Geometry check sheet. Reference: the model listing, model coordinates, mm. A direction names the side the tool comes from. Give positions to 0.01 mm unless a question says otherwise; leave off trailing zeros. Write each loop counter-clockwise with the first axis right and the second up, starting at its lowest first coordinate (ties: lowest second). Pieces come first, ordered by that corner, then holes. Notation, with made-up numbers: M 43,16 L 69,16 A20 cw 69,42 Z; hole C -6,31.25 d4. An arc over 180 degrees is marked long. Use one line per item in the form item = value. Start each with the question number.
Autodesk Inventor part; units mm, degrees
ref_plane "YZ Plane" through (0, 0, 0) normal (1, 0, 0) x (0, 1, 0)
ref_plane "XZ Plane" through (0, 0, 0) normal (0, 1, 0) x (-1, 0, 0)
ref_plane "XY Plane" through (0, 0, 0) normal (0, 0, 1) x (1, 0, 0)
sketch "Sketch1" plane through (0, 0, 0) normal (0, 0, 1) x (1, 0, 0)
  line L0 (0, 0) -> (25.4, 0)
  line L1 (25.4, 0) -> (25.4, 25.4)
  line L2 (25.4, 25.4) -> (0, 25.4)
  line L3 (0, 25.4) -> (0, 0)
  line L4 (1.5875, 23.8125) -> (23.8125, 23.8125)
  line L5 (23.8125, 23.8125) -> (23.8125, 1.5875)
  line L6 (23.8125, 1.5875) -> (1.5875, 1.5875)
  line L7 (1.5875, 1.5875) -> (1.5875, 23.8125)
  dimension "d0" = 25.4
  dimension "d2" = 25.4
  dimension "d3" = 1.5875
extrude "Extrusion1" add sketch "Sketch1" along normal blind 596.9
sketch "Sketch3" plane through (0, 0, 0) normal (0, -1, 0) x (1, 0, 0)
  circle A0 centre (12.7, 574.675) radius 3.3782
  circle A1 centre (12.7, 542.925) radius 3.3782
extrude "Extrusion3" cut sketch "Sketch3" against normal blind 25.4
sketch "Sketch4" plane through (0, 0, 0) normal (-1, 0, 0) x (0, 0, 1)
  circle A0 centre (533.4, 12.7) radius 3.3782
  circle A1 centre (584.2, 12.7) radius 3.3782
extrude "Extrusion4" cut sketch "Sketch4" against normal blind 25.4
sketch "Sketch5" plane through (25.4, 0, 0) normal (1, 0, 0) x (0, 0, -1)
  line L0 (0, 25.4) -> (-596.9, 25.4)
  line L1 (-596.9, 0) -> (-596.9, 25.4)
  circle A0 centre (-498.475, 12.7) radius 3.3782
  circle A1 centre (-304.8, 12.7) radius 3.3782
  circle A2 centre (-114.3, 12.7) radius 3.3782
  dimension "d12" = 6.7564
  dimension "d13" = 6.7564
  dimension "d14" = 98.425
  dimension "d15" = 292.1
  dimension "d16" = 6.7564
  dimension "d17" = 482.6
  dimension "d18" = 12.7
  dimension "d19" = 12.7
  dimension "d20" = 12.7
extrude "Extrusion5" cut sketch "Sketch5" against normal blind 25.4
properties part number "Inner Mount" material "Aluminum 6061"
(1) Depth check by flat-ended pin: pin 1 (12 mm diameter, centred on y = 21.5, z = 529.5, fed in from -X). Enter the tip coordinate at first touch or a pass-through.
(2) Draft check along Y on faces 3 (the flat face through (13, 0, 294)), 4 (the flat face through (1, 13, 596.9)), 5 (the flat face through (13, 23.812, 294)). Enter one of: released by +Y, released by -Y, zero draft, split by the parting line, or undercut.
(3) Sectioned sample at A-A, the plane x = 5.5. Record the boundary of the cut face in (y, z), plus the area to 3 significant figures.
(4) Tool access check on faces 1 (the flat face through (0, 13, 294)), 2 (the flat face through (23.812, 13, 294)). Record the directions out of +Z, -Z, +X, -X, +Y, -Y that give a thin tool (end or side, any length) a straight path to the whole face; none if there is none.
(5) Sectioned sample at B-B, the plane z = 358.5. Record the boundary of the cut face in (x, y).
(6) Thickness scan on probe 1 along Y at (x, z) = (3.5, 359); probe 2 along Z at (x, y) = (12.7, 0.45). Record the ranges inside material, lowest first. Write a range as [from, to].
Numbers:
q1.pin_1 = 0
q2.face_3 = released by -Y
q2.face_4 = zero draft
q2.face_5 = undercut
q3.outline = M 0,0 L 1.59,0 L 1.59,596.9 L 0,596.9 Z; M 23.81,0 L 25.4,0 L 25.4,596.9 L 23.81,596.9 Z
q3.area = 1,900 mm2
q4.face_1 = +Z, -Z, -X, +Y, -Y
q4.face_2 = +Z, -Z
q5.outline = M 0,0 L 25.4,0 L 25.4,25.4 L 0,25.4 Z; hole M 1.59,1.59 L 23.81,1.59 L 23.81,23.81 L 1.59,23.81 Z
q6.probe_1 = [0, 1.59], [23.81, 25.4]
q6.probe_2 = [0, 539.55], [546.3, 571.3], [578.05, 596.9]
